The model under review builds one solid part; all positions refer to its coordinate system, in mm. A direction names the side the tool comes from. Round coordinates to 2 decimals unless told otherwise and drop trailing zeros. Loops run counter-clockwise (first coordinate to the right, second up) from the corner with the lowest first, then second, coordinate; pieces in that order, holes last. Notation, with made-up numbers: (47.25, 3.5) -> (79.25, 3.5) arc R32 ccw to (79.25, 42.5) -> close; hole circle Ø8 at (38.5, 52). An arc over 180 degrees is marked (long way). Use a Markdown table: item, result. Add a question column.
1) Mouldability with a two-part tool opening along Y and no side actions: class faces 5 (the flat face through (0.7, 22, 19)), 6 (the flat face through (42, 0, 9)), 7 (the flat face through (42, 13, 2)) as released by +Y, released by -Y, zero draft, split by the parting line, or undercut.
2) Consider section C-C on z = 6.5. Give the boundary of the cut face in (x, y).
3) Consider section A-A on x = 14. Give the boundary of the cut face in (y, z) (3 decimals).
4) Insertion check: pin 1 (10 mm diameter, centred on x = 15, y = 5, fed in from +Z); pin 2 (0.6 mm diameter, centred on x = 43, y = 44.5, fed in from -Z); pin 3 (5 mm diameter, centred on x = 59, y = 40, fed in from +Z); pin 4 (1.5 mm diameter, centred on y = 21, z = 18.5, fed in from -X). Each pin has a flat end and moves straight along its axis. Give the tip position at first contact, or say it passes through.
5) Consider section B-B on y = 26.5. Give the boundary of the cut face in (x, z), plus the area to 3 significant figures.
6) Consider section D-D on y = 42.5. Give the boundary of the cut face in (x, z).
7) For faces 1 (the cylindrical face through (79.5, 36, 15.4)), 2 (the cylindrical face through (79.93, 34.532, 11.432)), 3 (the flat face through (21, 29, 8)), 4 (the flat face through (84.3, 22, 19)), list the 3-axis set-ups (+Z, -Z, +X, -X, +Y, -Y) from which the entire face can be reached by the end or side of a thin tool; tool diameter is ignored.
8) Wall thickness on probe 1 along Y at (x, z) = (79.25, 12.4); probe 2 along X at (y, z) = (43.5, 12.25); probe 3 along Y at (x, z) = (16, 18.5): over which ranges is each line inside the solid? List them lowest first.
from build123d import *

# Parameters (mm, degrees)
SKETCH_1_W          = 85
SKETCH_1_H          = 45
EXTRUDE_1_DEPTH     = 20
SKETCH_2_W          = 82.6
SKETCH_2_H          = 42.6
CUT_EXTRUDE_1_DEPTH = 18
SKETCH_3_R          = 52.564832307
SKETCH_3_W          = 83.6
SKETCH_3_H          = 43.6
CUT_EXTRUDE_2_DEPTH = 3
SKETCH_4_R          = 1.5
CUT_EXTRUDE_3_DEPTH = 10
SKETCH_6_R          = 1.5
EXTRUDE_2_DEPTH     = 6
SKETCH_7_R          = 0.65
EXTRUDE_3_DEPTH     = 2
SKETCH_5_W          = 28
SKETCH_5_H          = 15.9
CUT_EXTRUDE_4_DEPTH = 99.234413522
SKETCH_9_W          = 32
SKETCH_9_H          = 19.9
CUT_EXTRUDE_5_DEPTH = 1
SKETCH_10_W         = 14.5
SKETCH_10_H         = 8
SKETCH_10_W_2       = 7.8
SKETCH_10_H_2       = 4
CUT_EXTRUDE_6_DEPTH = 10
FILLET_1_R          = 1
SKETCH_11_R         = 1.8
EXTRUDE_4_DEPTH     = 10
SKETCH_12_R         = 1.8
CUT_EXTRUDE_7_DEPTH = 90.721792225
SKETCH_13_R         = 2.425
CUT_EXTRUDE_8_DEPTH = 98.846819059


with BuildPart() as part:
    # Эскиз1 → Бобышка-Вытянуть1 (new body)
    with BuildSketch(Plane.XY):
        with Locations((42.5, 22.5)):
            Rectangle(SKETCH_1_W, SKETCH_1_H)
    extrude(amount=EXTRUDE_1_DEPTH)

    # Эскиз2 → Вырез-Вытянуть1 (cut)
    with BuildSketch(Plane.XY.offset(20)):
        with Locations((42.5, 22.5)):
            Rectangle(SKETCH_2_W, SKETCH_2_H)
    extrude(amount=-CUT_EXTRUDE_1_DEPTH, mode=Mode.SUBTRACT)

    # Эскиз3 → Вырез-Вытянуть2 (cut)
    with BuildSketch(Plane.XY.offset(20)):
        with Locations((42.5, 22.5)):
            Circle(SKETCH_3_R)
        with Locations((42.5, 22.5)):
            Rectangle(SKETCH_3_W, SKETCH_3_H, mode=Mode.SUBTRACT)
    extrude(amount=-CUT_EXTRUDE_2_DEPTH, mode=Mode.SUBTRACT)

    # Эскиз4 → Вырез-Вытянуть3 (cut)
    with BuildSketch(Plane.ZY.offset(-85)):
        with Locations(Location((12.4, 36.05, 0), (0, 0, 180))):
            Circle(SKETCH_4_R)
    extrude(amount=CUT_EXTRUDE_3_DEPTH, mode=Mode.SUBTRACT)

    # Эскиз6 → Бобышка-Вытянуть2 (add)
    with BuildSketch(Plane.XY.offset(2)):
        with Locations((21, 29.89)):
            Circle(SKETCH_6_R)
        with Locations((63.5, 32)):
            Circle(SKETCH_6_R)
    extrude(amount=EXTRUDE_2_DEPTH)

    # Эскиз7 → Бобышка-Вытянуть3 (add)
    with BuildSketch(Plane.XY.offset(8)):
        with Locations((21, 29.89)):
            Circle(SKETCH_7_R)
        with Locations((63.5, 32)):
            Circle(SKETCH_7_R)
    extrude(amount=EXTRUDE_3_DEPTH)

    # Эскиз5 → Вырез-Вытянуть4 (cut, through all)
    with BuildSketch(Plane(origin=(0, 0, 0), x_dir=(-1, 0, 0), z_dir=(0, 0, -1))):
        with Locations((-41.8, 24.64)):
            Rectangle(SKETCH_5_W, SKETCH_5_H)
    extrude(amount=-CUT_EXTRUDE_4_DEPTH, mode=Mode.SUBTRACT)

    # Эскиз9 → Вырез-Вытянуть5 (cut)
    with BuildSketch(Plane.XY.offset(2)):
        with Locations((41.8, 24.64)):
            Rectangle(SKETCH_9_W, SKETCH_9_H)
    extrude(amount=-CUT_EXTRUDE_5_DEPTH, mode=Mode.SUBTRACT)

    # Эскиз10 → Вырез-Вытянуть6 (cut)
    with BuildSketch(Plane.XZ.offset(-45)):
        with Locations((29.85, 12)):
            Rectangle(SKETCH_10_W, SKETCH_10_H)
        with Locations((55.15, 12)):
            Rectangle(SKETCH_10_W, SKETCH_10_H)
        with Locations((42.5, 10.5)):
            Rectangle(SKETCH_10_W_2, SKETCH_10_H_2)
    extrude(amount=CUT_EXTRUDE_6_DEPTH, mode=Mode.SUBTRACT)

    # Скругление1
    fillet_1_edges = [part.edges().sort_by_distance(p)[0] for p in [
        (0, 45, 8.5),
        (85, 45, 8.5),
        (85, 0, 8.5),
        (0, 0, 8.5),
        (42.5, 45, 0),
        (85, 22.5, 0),
        (42.5, 0, 0),
        (0, 22.5, 0),
    ]]
    fillet(fillet_1_edges, radius=FILLET_1_R)

    # Эскиз11 → Бобышка-Вытянуть4 (add)
    with BuildSketch(Plane.ZY.offset(-85)):
        with BuildLine():
            Line((1, 37.8), (1, 34.3))
            Line((1, 34.3), (10.741687605, 33.55))
            ThreePointArc((10.741687605, 33.55), (15.4, 36.05), (10.741687605, 38.55))
            Line((10.741687605, 38.55), (1, 37.8))
        make_face()
        with Locations(Location((12.4, 36.05, 0), (0, 0, 180))):
            Circle(SKETCH_11_R, mode=Mode.SUBTRACT)
    extrude(amount=EXTRUDE_4_DEPTH)

    # Эскиз12 → Вырез-Вытянуть7 (cut, through all)
    with BuildSketch(Plane.ZY.offset(-75)):
        with Locations(Location((12.4, 36.05, 0), (0, 0, 180))):
            Circle(SKETCH_12_R)
    extrude(amount=-CUT_EXTRUDE_7_DEPTH, mode=Mode.SUBTRACT)

    # Эскиз13 → Вырез-Вытянуть8 (cut, through all)
    with BuildSketch(Plane.XY.offset(2)):
        with Locations((14, 36.89)):
            Circle(SKETCH_13_R)
    extrude(amount=-CUT_EXTRUDE_8_DEPTH, mode=Mode.SUBTRACT)


solid = part.part
Result set:
| question | item | result |
|---|---|---|
| 1 | face 5 | zero draft |
| 1 | face 6 | released by -Y |
| 1 | face 7 | undercut |
| 2 | outline | (0, 1) arc R1 ccw to (1, 0) -> (84, 0) arc R1 ccw to (85, 1) -> (85, 44) arc R1 ccw to (84, 45) -> (1, 45) arc R1 ccw to (0, 44) -> close; circle Ø3 at (21, 29.89); circle Ø3 at (63.5, 32); hole (1.2, 1.2) -> (83.8, 1.2) -> (83.8, 33.88) -> (75, 33.88) -> (75, 38.22) -> (83.8, 38.22) -> (83.8, 43.8) -> (1.2, 43.8) -> close |
| 3 | outline | (0, 1) arc R1 ccw to (1, 0) -> (34.465, 0) -> (34.465, 2) -> (1.2, 2) -> (1.2, 20) -> (0.7, 20) -> (0.7, 17) -> (0, 17) -> close; (39.315, 0) -> (44, 0) arc R1 ccw to (45, 1) -> (45, 17) -> (44.3, 17) -> (44.3, 20) -> (43.8, 20) -> (43.8, 2) -> (39.315, 2) -> close |
| 4 | pin 1 | z = 20 |
| 4 | pin 2 | z = 0.02 |
| 4 | pin 3 | z = 2 |
| 4 | pin 4 | x = 0.7 |
| 5 | outline | (0, 1) arc R1 ccw to (1, 0) -> (27.8, 0) -> (27.8, 1) -> (25.8, 1) -> (25.8, 2) -> (1.2, 2) -> (1.2, 20) -> (0.7, 20) -> (0.7, 17) -> (0, 17) -> close; (55.8, 0) -> (84, 0) arc R1 ccw to (85, 1) -> (85, 17) -> (84.3, 17) -> (84.3, 20) -> (83.8, 20) -> (83.8, 2) -> (57.8, 2) -> (57.8, 1) -> (55.8, 1) -> close |
| 5 | area | 149 mm2 |
| 6 | outline | (0, 1) arc R1 ccw to (1, 0) -> (84, 0) arc R1 ccw to (85, 1) -> (85, 17) -> (84.3, 17) -> (84.3, 20) -> (83.8, 20) -> (83.8, 2) -> (1.2, 2) -> (1.2, 20) -> (0.7, 20) -> (0.7, 17) -> (0, 17) -> close |
| 7 | face 1 | none |
| 7 | face 2 | +X |
| 7 | face 3 | +Z |
| 7 | face 4 | +Z, +X, +Y, -Y |
| 8 | probe 1 | 0 to 1.2, 33.05 to 34.25, 37.85 to 39.05, 43.8 to 45 |
| 8 | probe 2 | 0 to 1.2, 83.8 to 85 |
| 8 | probe 3 | 0.7 to 1.2, 43.8 to 44.3 |
